```python
from build123d import *

# Parameters (mm, degrees)
SKETCH_1_W          = 200
SKETCH_1_H          = 200
SKETCH_1_R          = 12.5
EXTRUDE_1_DEPTH     = 5
SKETCH_3_R          = 2.5
CUT_EXTRUDE_2_DEPTH = 142.509716981
SKETCH_4_R          = 2.55
SKETCH_4_R_2        = 7.5
CUT_EXTRUDE_3_DEPTH = 142.509716981
CUT_EXTRUDE_4_DEPTH = 142.509716981


with BuildPart() as part:
    # ｽｹｯﾁ1 → ﾎﾞｽ - 押し出し1 (new body)
    with BuildSketch(Plane.XY):
        Rectangle(SKETCH_1_W, SKETCH_1_H)
        Circle(SKETCH_1_R, mode=Mode.SUBTRACT)
    extrude(amount=EXTRUDE_1_DEPTH)

    # ｽｹｯﾁ3 → ｶｯﾄ - 押し出し2 (cut, through all)
    with BuildSketch(Plane.XY.offset(5)):
        with Locations((0, 90)):
            Circle(SKETCH_3_R)
        with Locations((90, 90)):
            Circle(SKETCH_3_R)
        with Locations((-90, 90)):
            Circle(SKETCH_3_R)
        with Locations((-90, -90)):
            Circle(SKETCH_3_R)
        with Locations((0, -90)):
            Circle(SKETCH_3_R)
        with Locations((90, -90)):
            Circle(SKETCH_3_R)
    extrude(amount=-CUT_EXTRUDE_2_DEPTH, mode=Mode.SUBTRACT)

    # ｽｹｯﾁ4 → ｶｯﾄ - 押し出し3 (cut, through all)
    with BuildSketch(Plane.XY.offset(5)):
        with Locations((0, 30)):
            Circle(SKETCH_4_R)
        with Locations((25.980762114, 15)):
            Circle(SKETCH_4_R)
        with Locations((25.980762114, -15)):
            Circle(SKETCH_4_R)
        with Locations((0, -30)):
            Circle(SKETCH_4_R)
        with Locations((-25.980762114, -15)):
            Circle(SKETCH_4_R)
        with Locations((-25.980762114, 15)):
            Circle(SKETCH_4_R)
        with Locations((-75, 0)):
            Circle(SKETCH_4_R_2)
        with Locations(Location((75, 0, 0), (0, 0, 180))):
            Circle(SKETCH_4_R_2)
    extrude(amount=-CUT_EXTRUDE_3_DEPTH, mode=Mode.SUBTRACT)

    # ｽｹｯﾁ5 → ｶｯﾄ - 押し出し4 (cut, through all)
    with BuildSketch(Plane.XY.offset(5)):
        with BuildLine():
            Line((-80, 70), (-80, 25))
            ThreePointArc((-80, 25), (-77.071067812, 17.928932188), (-70, 15))
            Line((-70, 15), (-48.989794856, 15))
            ThreePointArc((-48.989794856, 15), (-43.767465177, 16.471971346), (-40.082559427, 20.454545455))
            ThreePointArc((-40.082559427, 20.454545455), (-31.819805153, 31.819805153), (-20.454545455, 40.082559427))
            ThreePointArc((-20.454545455, 40.082559427), (-16.471971346, 43.767465177), (-15, 48.989794856))
            Line((-15, 48.989794856), (-15, 70))
            ThreePointArc((-15, 70), (-17.928932188, 77.071067812), (-25, 80))
            Line((-25, 80), (-70, 80))
            ThreePointArc((-70, 80), (-77.071067812, 77.071067812), (-80, 70))
        make_face()
        with BuildLine():
            Line((15, 48.989794856), (15, 70))
            ThreePointArc((15, 70), (17.928932188, 77.071067812), (25, 80))
            Line((25, 80), (70, 80))
            ThreePointArc((70, 80), (77.071067812, 77.071067812), (80, 70))
            Line((80, 70), (80, 25))
            ThreePointArc((80, 25), (77.071067812, 17.928932188), (70, 15))
            Line((70, 15), (48.989794856, 15))
            ThreePointArc((48.989794856, 15), (43.767465177, 16.471971346), (40.082559427, 20.454545455))
            ThreePointArc((40.082559427, 20.454545455), (31.819805153, 31.819805153), (20.454545455, 40.082559427))
            ThreePointArc((20.454545455, 40.082559427), (16.471971346, 43.767465177), (15, 48.989794856))
        make_face()
        with BuildLine():
            Line((15, -48.989794856), (15, -70))
            ThreePointArc((15, -70), (17.928932188, -77.071067812), (25, -80))
            Line((25, -80), (70, -80))
            ThreePointArc((70, -80), (77.071067812, -77.071067812), (80, -70))
            Line((80, -70), (80, -25))
            ThreePointArc((80, -25), (77.071067812, -17.928932188), (70, -15))
            Line((70, -15), (48.989794856, -15))
            ThreePointArc((48.989794856, -15), (43.767465177, -16.471971346), (40.082559427, -20.454545455))
            ThreePointArc((40.082559427, -20.454545455), (31.819805153, -31.819805153), (20.454545455, -40.082559427))
            ThreePointArc((20.454545455, -40.082559427), (16.471971346, -43.767465177), (15, -48.989794856))
        make_face()
        with BuildLine():
            Line((-15, -48.989794856), (-15, -70))
            ThreePointArc((-15, -70), (-17.928932188, -77.071067812), (-25, -80))
            Line((-25, -80), (-70, -80))
            ThreePointArc((-70, -80), (-77.071067812, -77.071067812), (-80, -70))
            Line((-80, -70), (-80, -25))
            ThreePointArc((-80, -25), (-77.071067812, -17.928932188), (-70, -15))
            Line((-70, -15), (-48.989794856, -15))
            ThreePointArc((-48.989794856, -15), (-43.767465177, -16.471971346), (-40.082559427, -20.454545455))
            ThreePointArc((-40.082559427, -20.454545455), (-31.819805153, -31.819805153), (-20.454545455, -40.082559427))
            ThreePointArc((-20.454545455, -40.082559427), (-16.471971346, -43.767465177), (-15, -48.989794856))
        make_face()
    extrude(amount=-CUT_EXTRUDE_4_DEPTH, mode=Mode.SUBTRACT)


solid = part.part
```
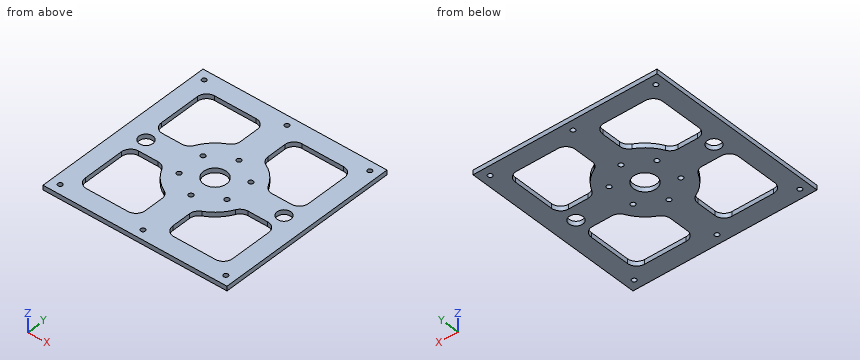
Source: CAD feature listing. Evaluate the final solid. Frame: model axes, mm. Coordinates: 2 decimals unless noted, no trailing zeros. Loops run counter-clockwise (first coordinate to the right, second up) from the corner with the lowest first, then second, coordinate; pieces in that order, holes last. Notation, with made-up numbers: M 83.25,13 L 132.25,13 A24 cw 132.25,39 Z; hole C 76,42.5 d4. An arc over 180 degrees is marked long. Use a Markdown table: item, result. Add a question column.
Q1. Section query C-C, the plane x = -90. Return loops of the section in (y, z).
Q2. Section query D-D, the plane y = 0. Return loops of the section in (x, z), and give its area (3 significant figures).
Q3. Section query B-B, the plane x = 0. Return loops of the section in (y, z), and give its area (3 significant figures).
Q4. First-contact query: pin 1 (8 mm diameter, centred on x = 0, y = -30, fed in from +Z); pin 2 (3 mm diameter, centred on x = 90, y = -90, fed in from +Z). Flat tips, straight axial feed; report the tip coordinate or a pass-through.
Q5. Material intervals for L1, parallel to Y at x = 0, z = 1.85; L2, parallel to Y at x = 90, z = 1.85; L3, parallel to X at y = 89.5, z = 4.45, sorted ascending.
Q6. Section query A-A, the plane y = 90. Return loops of the section in (x, z), and give its area (3 significant figures).
Result:
| question | item | result |
|---|---|---|
| 1 | outline | M -100,0 L -92.5,0 L -92.5,5 L -100,5 Z; M -87.5,0 L 87.5,0 L 87.5,5 L -87.5,5 Z; M 92.5,0 L 100,0 L 100,5 L 92.5,5 Z |
| 2 | outline | M -100,0 L -82.5,0 L -82.5,5 L -100,5 Z; M -67.5,0 L -12.5,0 L -12.5,5 L -67.5,5 Z; M 12.5,0 L 67.5,0 L 67.5,5 L 12.5,5 Z; M 82.5,0 L 100,0 L 100,5 L 82.5,5 Z |
| 2 | area | 725 mm2 |
| 3 | outline | M -100,0 L -92.5,0 L -92.5,5 L -100,5 Z; M -87.5,0 L -32.55,0 L -32.55,5 L -87.5,5 Z; M -27.45,0 L -12.5,0 L -12.5,5 L -27.45,5 Z; M 12.5,0 L 27.45,0 L 27.45,5 L 12.5,5 Z; M 32.55,0 L 87.5,0 L 87.5,5 L 32.55,5 Z; M 92.5,0 L 100,0 L 100,5 L 92.5,5 Z |
| 3 | area | 774 mm2 |
| 4 | pin 1 | stops at z = 5 |
| 4 | pin 2 | passes through |
| 5 | L1 | y = -100 to -92.5, -87.5 to -32.55, -27.45 to -12.5, 12.5 to 27.45, 32.55 to 87.5, 92.5 to 100 |
| 5 | L2 | y = -100 to -92.5, -87.5 to 87.5, 92.5 to 100 |
| 5 | L3 | x = -100 to -92.45, -87.55 to -2.45, 2.45 to 87.55, 92.45 to 100 |
| 6 | outline | M -100,0 L -92.5,0 L -92.5,5 L -100,5 Z; M -87.5,0 L -2.5,0 L -2.5,5 L -87.5,5 Z; M 2.5,0 L 87.5,0 L 87.5,5 L 2.5,5 Z; M 92.5,0 L 100,0 L 100,5 L 92.5,5 Z |
| 6 | area | 925 mm2 |
